from build123d import *

# Parameters (mm, degrees)
BOSS_EXTRUDE1_DEPTH = 15.9512
FILLET1_R           = 2.54
SKETCH3_R           = 2.38125
CUT_EXTRUDE1_DEPTH  = 60.67865116


with BuildPart() as part:
    # Sketch2 → Boss-Extrude1 (new body)
    with BuildSketch(Plane(origin=(0, 0, 0), x_dir=(1, 0, 0), z_dir=(0, 1, 0))):
        with BuildLine():
            Line((-43.856127716, 39.498822447), (-43.856127716, 7.240822447))
            ThreePointArc((-43.856127716, 7.240822447), (-37.287152217, 2.576192047), (-35.048092212, 10.315496032))
            ThreePointArc((-35.048092212, 10.315496032), (-36.919453616, 27.093420789), (-22.621727716, 36.069822447))
            Line((-22.621727716, 36.069822447), (-22.621727716, 39.498822447))
            Line((-22.621727716, 39.498822447), (-43.856127716, 39.498822447))
        make_face()
        with BuildLine():
            Line((-1.387327716, 39.498822447), (-22.621727716, 39.498822447))
            Line((-22.621727716, 39.498822447), (-22.621727716, 36.069822447))
            ThreePointArc((-22.621727716, 36.069822447), (-8.324001816, 27.093420789), (-10.19536322, 10.315496032))
            ThreePointArc((-10.19536322, 10.315496032), (-7.956303215, 2.576192047), (-1.387327716, 7.240822447))
            Line((-1.387327716, 7.240822447), (-1.387327716, 39.498822447))
        make_face()
    extrude(amount=BOSS_EXTRUDE1_DEPTH)

    # Fillet1
    fillet1_edges = [part.edges().sort_by_distance(p)[0] for p in [
        (-43.856127716, 7.9756, -39.498822447),
        (-1.387327716, 7.9756, -39.498822447),
    ]]
    fillet(fillet1_edges, radius=FILLET1_R)

    # Sketch3 → Cut-Extrude1 (cut, through all)
    with BuildSketch(Plane(origin=(0, 0, -39.498822447), x_dir=(-1, 0, 0), z_dir=(0, 0, -1))):
        with Locations((22.621727716, 7.9756)):
            Circle(SKETCH3_R)
    extrude(amount=-CUT_EXTRUDE1_DEPTH, mode=Mode.SUBTRACT)


solid = part.part
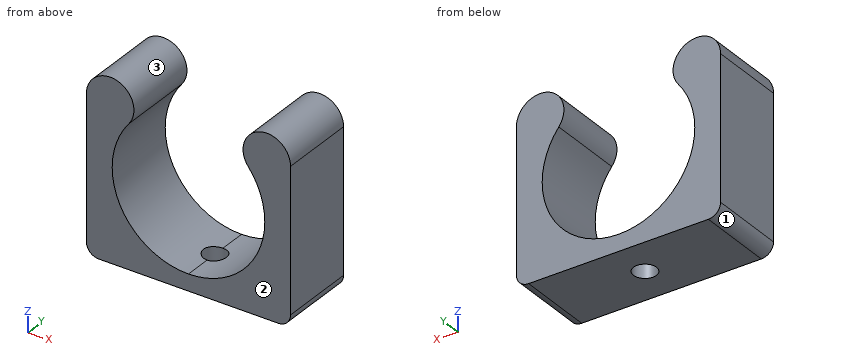
Work out the finished part from the listing and answer in its coordinate system (mm). Face numbers are marked on the shaded views. Give positions to 0.01 mm unless a question says otherwise; leave off trailing zeros. Write each loop counter-clockwise with the first axis right and the second up, starting at its lowest first coordinate (ties: lowest second). Pieces come first, ordered by that corner, then holes.
Q1. For a pull along Z with two mould halves and no side action, classify the marked faces 1, 2 and 3 as released by +Z, released by -Z, zero draft, split by the parting line, or undercut.
Answer:
face 1: released by -Z
face 2: zero draft
face 3: undercut
Q2. The part is cut by section B-B on x = -24. Give the vertices of the cut face in (y, z), and give its area (3 significant figures).
Answer:
outline: (0, -39.5) - (6.03, -39.5) - (6.03, -36.01) - (0, -36.01) - close; (9.92, -39.5) - (15.95, -39.5) - (15.95, -36.01) - (9.92, -36.01) - close
area: 42.1 mm2
Q3. The part is cut by section D-D on x = -18. Give the vertices of the cut face in (y, z).
Answer:
outline: (0, -39.5) - (15.95, -39.5) - (15.95, -35.38) - (0, -35.38) - close
Q4. Straight lines are drawn through the part: L1, parallel to X at y = 9.75, z = -13.5; L2, parallel to X at y = 2.5, z = -16; L3, parallel to Z at x = -8, y = 4.75. For each, find the intervals that lie inside material, in ascending order.
Answer:
L1: x = -43.86 to -37.02, -8.23 to -1.39
L2: x = -43.86 to -37.93, -7.31 to -1.39
L3: z = -39.5 to -26.38, -14.01 to -2.59
Q5. The part is cut by section A-A on z = -33. Give the vertices of the cut face in (x, y).
Answer:
outline: (-43.86, 0) - (-32, 0) - (-32, 15.95) - (-43.86, 15.95) - close; (-13.24, 0) - (-1.39, 0) - (-1.39, 15.95) - (-13.24, 15.95) - close
